Autodesk Inventor part; units mm, degrees
ref_plane "YZ Plane" through (0, 0, 0) normal (1, 0, 0) x (0, 1, 0)
ref_plane "XZ Plane" through (0, 0, 0) normal (0, 1, 0) x (-1, 0, 0)
ref_plane "XY Plane" through (0, 0, 0) normal (0, 0, 1) x (1, 0, 0)
sketch "Sketch1" plane through (0, 0, 0) normal (0, 0, 1) x (1, 0, 0)
  circle A0 centre (0, 0) radius 2.5
  circle A1 centre (0, 0) radius 12
  circle A2 centre (0, 0) radius 7.95
  dimension "d0" = 5
  dimension "d1" = 24
  dimension "d2" = 15.9
extrude "Extrusion1" add sketch "Sketch1" along normal mid plane 11 contours A2
extrude "Extrusion2" add sketch "Sketch1" along normal mid plane 10.3 contours A1
chamfer "Chamfer1" distance 2.5 angle 45 2 edges at (-12, 0, 5.15) (-12, 0, -5.15)
properties part number "Printer Wheel"
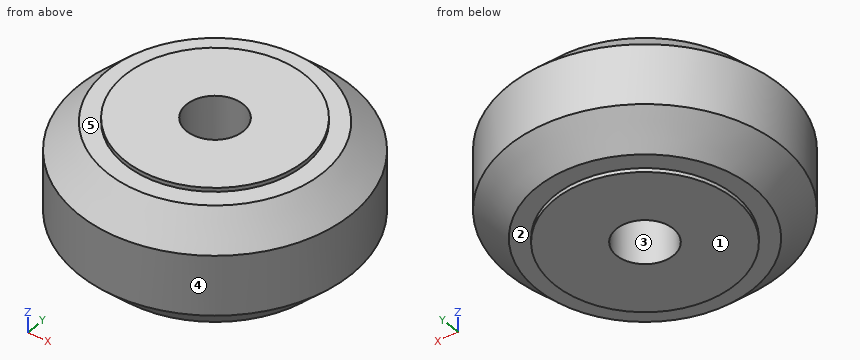
Design review of the part built by this model. Coordinates are the model's own, in mm. Face numbers are marked on the shaded views. A direction names the side the tool comes from. Coordinates: 2 decimals unless noted, no trailing zeros. Loops run counter-clockwise (first coordinate to the right, second up) from the corner with the lowest first, then second, coordinate; pieces in that order, holes last.
Q1. The part is to be moulded in two halves that separate along Y. For the marked faces 3, 4 and 5, say which applies: +Y half, -Y half, draft (parallel to the pull), parting line (faces both ways), or undercut.
Reported:
face 3: undercut
face 4: parting line
face 5: draft
Q2. We need section A-A on x = 0. State the section outline as (y, z) points.
Reported:
outline: (-12, -2.65) - (-9.5, -5.15) - (-7.95, -5.15) - (-7.95, -5.5) - (-2.5, -5.5) - (-2.5, 5.5) - (-7.95, 5.5) - (-7.95, 5.15) - (-9.5, 5.15) - (-12, 2.65) - close; (2.5, -5.5) - (7.95, -5.5) - (7.95, -5.15) - (9.5, -5.15) - (12, -2.65) - (12, 2.65) - (9.5, 5.15) - (7.95, 5.15) - (7.95, 5.5) - (2.5, 5.5) - close
Q3. Tool access review of the marked faces 1 and 2: name each direction out of +Z, -Z, +X, -X, +Y, -Y from which nothing blocks a thin tool from reaching the whole face with its end or side.
Reported:
face 1: -Z, +X, -X, +Y, -Y
face 2: -Z
Q4. For pin 1 (4 mm diameter, centred on x = 3.5, z = 3.5, fed in from -Y); pin 2 (1.5 mm diameter, centred on y = 7.5, z = 3, fed in from +X); pin 3 (6 mm diameter, centred on x = 5, z = -2.5, fed in from +Y), all flat-tipped, find the tip position at first contact; note any pin that passes through.
Reported:
pin 1: stops at y = -11.88
pin 2: stops at x = 9.86
pin 3: stops at y = 11.83
Q5. To check wall thickness, follow line 1 (Y direction, x = 0, z = -2.5); line 2 (Y direction, x = -2, z = 3.5); line 3 (Z direction, x = -6.5, y = -5.25). State the ranges of each line that lie inside material, in increasing order.
Reported:
line 1: y = -12 to -2.5, 2.5 to 12
line 2: y = -10.97 to -1.5, 1.5 to 10.97
line 3: z = -5.15 to 5.15
Q6. We need section C-C on z = 1.75. State the section outline as (x, y) points.
Reported:
outline: circle Ø24 at (0, 0); hole circle Ø5 at (0, 0)
